The model under review builds one solid part; all positions refer to its coordinate system, in mm. Face numbers are marked on the shaded views. A direction names the side the tool comes from. Give positions to 0.01 mm unless a question says otherwise; leave off trailing zeros. Write each loop counter-clockwise with the first axis right and the second up, starting at its lowest first coordinate (ties: lowest second). Pieces come first, ordered by that corner, then holes.
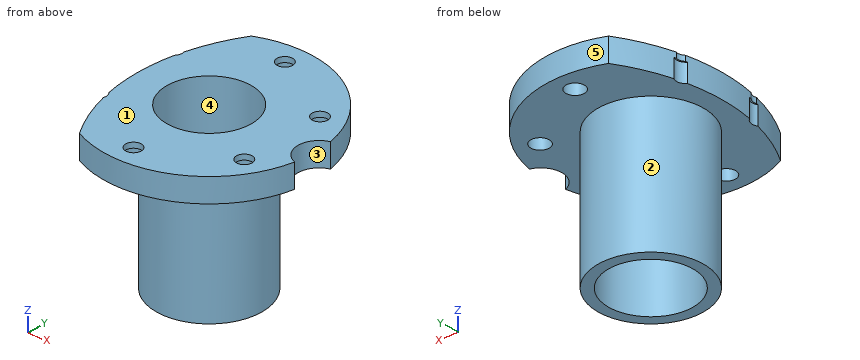
Autodesk Inventor part; units mm, degrees
ref_plane "YZ Plane" through (0, 0, 0) normal (1, 0, 0) x (0, 1, 0)
ref_plane "XZ Plane" through (0, 0, 0) normal (0, 1, 0) x (-1, 0, 0)
ref_plane "XY Plane" through (0, 0, 0) normal (0, 0, 1) x (1, 0, 0)
sketch "Sketch1" plane through (0, 0, 0) normal (0, 0, 1) x (1, 0, 0)
  circle A0 centre (0, 0) radius 15.875
  circle A1 centre (0, 0) radius 12.7
  dimension "d0" = 31.75
  dimension "d1" = 25.4
extrude "Eyepiece Extrusion" add sketch "Sketch1" against normal blind 40.64
sketch "Sketch2" plane through (0, 0, 0) normal (0, 0, 1) x (1, 0, 0)
  circle A0 centre (0, 0) radius 12.7
  circle A1 centre (0, 0) radius 31.75
  dimension "d6" = 25.4
  dimension "d7" = 63.5
extrude "Bolt Extrusion" add sketch "Sketch2" along normal blind 7.1374
sketch "Sketch3" plane through (0, 0, 0) normal (0, 0, -1) x (-1, 0, 0)
  circle A0 centre (0, 0) radius 31.75
  circle A1 centre (-33.1656, 0) radius 54.6286
  circle A2 centre (0, 0) radius 12.7
  circle A3 centre (0, 0) radius 15.875
  arc A4 (18.442, -17.4658) -> (18.442, 17.4658) centre (-33.1656, 0) ccw
  circle A5 centre (0, 0) radius 25.4 construction
  point P0 (13.2104, 28.8712)
  point P1 (13.2104, -28.8712)
  dimension "d8" = 108.966
extrude "Cutout For Filter Wheel" cut sketch "Sketch3" against normal through all contours A0 A1 picked at (24.3045, -5.7561)
sketch "Sketch8" plane through (0, 0, 7.1374) normal (0, 0, 1) x (1, 0, 0)
  circle A0 centre (33.1724, 0) radius 6.35
  point P0 (0, 0)
  dimension "d50" = 12.7
  dimension "d51" = 33.1724
extrude "Extrusion4" cut sketch "Sketch8" against normal through all
sketch "Sketch9" plane through (0, 0, 0) normal (0, 0, -1) x (-1, 0, 0)
  point P0 (0, 0)
  point P1 (0, 25.4)
  dimension "d59" = 25.4
hole "Hole4" at (0, 25.4, 0) direction (0, 0, 1) diameter 4.699 depth 7.1374 counterbore diameter 5.5372 counterbore depth 5.5524
pattern_circular "Circular Pattern2" count 6 over 360 about axis through (0, 0, -10) along (0, 0, 1) of "Hole4"
equation "\"d0\" = outsideDiameter"
equation "\"d1\" = insideDiameter"
equation "\"d2\" = extrusionNoseDepth"
equation "\"d6\" = insideDiameter"
equation "\"d7\" = maxOutsideDiameter"
equation "\"d4\" = support"
equation "\"outsideDiameter\" = 31.75"
equation "\"insideDiameter\" = 25.4"
equation "\"support\" = 7.1374"
equation "\"totalHeight\" = 44.45"
equation "\"maxOutsideDiameter\" = 63.5"
equation "\"eyepieceNoseDepth\" = 38.1"
equation "\"baseDepth\" = 2.54"
equation "\"extrusionNoseDepth\" = eyepieceNoseDepth + baseDepth"
equation "\"radiusForHoles\" = 25.4"
properties part number "insertToScope" material "PET Plastic"
1) Consider section D-D, the plane z = 1. Give the boundary of the cut face in (x, y), then the cut area to 3 significant figures.
2) Consider section C-C, the plane x = 0. State how many separate pieces and enclosed holes the cut face has, then the cut area to 3 significant figures.
3) Tool access review of the marked faces 1 and 2: name each direction out of +Z, -Z, +X, -X, +Y, -Y from which nothing blocks a thin tool from reaching the whole face with its end or side.
4) The part is to be moulded in two halves that separate along X. For the marked faces 3, 4 and 5, say which applies: +X half, -X half, draft (parallel to the pull), parting line (faces both ways), or undercut.
5) To check wall thickness, follow probe 1 along Y at (x, z) = (0, -28) (3 decimals); probe 2 along Z at (x, y) = (26, -8); probe 3 along Y at (x, z) = (1, -36.5). State the ranges of each line that lie inside material, in increasing order.
6) Insertion check: pin 1 (6 mm diameter, centred on x = 0, y = -24, fed in from -Z); pin 2 (5 mm diameter, centred on x = 12, z = -29.5, fed in from +Y); pin 3 (4 mm diameter, centred on x = 22, y = 12.7, fed in from -Z) (3 decimals); pin 4 (12 mm diameter, centred on y = -6.5, z = -26.5, fed in from -X). Each pin has a flat end and moves straight along its axis. Give the tip position at first contact, or say it passes through.
7) Consider section A-A, the plane y = 0. Give the boundary of the cut face in (x, z) (3 decimals), then the cut area to 3 significant figures.
8) Consider section B-B, the plane x = -8. Give the boundary of the cut face in (y, z).
Answer block:
1. outline: (-20.47, -10.39) arc R2.77 cw to (-19.61, -14.1) arc R54.63 ccw to (-13.21, -28.87) arc R31.75 ccw to (31.17, -6.03) arc R6.35 cw to (31.17, 6.03) arc R31.75 ccw to (-13.21, 28.87) arc R54.63 ccw to (-19.61, 14.1) arc R2.77 cw to (-20.47, 10.39) arc R54.63 ccw to start; hole circle Ø25.4 at (0, 0); hole circle Ø5.54 at (0, -25.4); hole circle Ø5.54 at (0, 25.4); hole circle Ø5.54 at (22, -12.7); hole circle Ø5.54 at (22, 12.7)
1. area: 2,070 mm2
2. separate pieces: 4
2. enclosed holes: 0
2. area: 454 mm2
3. face 1: +Z, +X, -X, +Y, -Y
3. face 2: -Z
4. face 3: +X half
4. face 4: undercut
4. face 5: parting line
5. probe 1: y = -15.875 to -12.7, 12.7 to 15.875
5. probe 2: z = 0 to 7.14
5. probe 3: y = -15.84 to -12.66, 12.66 to 15.84
6. pin 1: stops at z = 0
6. pin 2: stops at y = 12.72
6. pin 3: passes through
6. pin 4: stops at x = -15.87
7. outline: (-21.463, 0) - (-15.875, 0) - (-15.875, -40.64) - (-12.7, -40.64) - (-12.7, 7.137) - (-21.463, 7.137) - close; (12.7, -40.64) - (15.875, -40.64) - (15.875, 0) - (26.822, 0) - (26.822, 7.137) - (12.7, 7.137) - close
7. area: 421 mm2
8. outline: (-30.73, 0) - (-13.71, 0) - (-13.71, -40.64) - (-9.86, -40.64) - (-9.86, 7.14) - (-30.73, 7.14) - close; (9.86, -40.64) - (13.71, -40.64) - (13.71, 0) - (30.73, 0) - (30.73, 7.14) - (9.86, 7.14) - close
